Verification items for the finished model (mm, model axes). Round coordinates to 2 decimals unless told otherwise and drop trailing zeros. Write each loop counter-clockwise with the first axis right and the second up, starting at its lowest first coordinate (ties: lowest second). Pieces come first, ordered by that corner, then holes. Notation, with made-up numbers: (31.5, 74.25) - (38.5, 74.25) arc R23 ccw to (38.5, 99.25) - close; hole circle Ø10 at (67, 66). An arc over 180 degrees is marked (long way). Answer as a JSON object with one key per item and string values. Group by question number.
1) Thickness scan on line 1 (Y direction, x = 3, z = 2.25); line 2 (X direction, y = 1.65, z = -2.25); line 3 (Z direction, x = 9.5, y = 0.25). Record the ranges inside material, lowest first.
2) Section check D-D (x = -10). Enter the section's corners in (y, z).
3) Go/stop test with flat-tipped pins: pin 1 Ø4 at (x, z) = (-6, -1.5) entering from +Y; pin 2 Ø3 at (x, z) = (0, 0) entering from +Y. Record where each tip stops, or that it passes through.
4) Section check B-B (y = 0.65). State how many separate pieces and enclosed holes the cut face has, then the cut area to 3 significant figures.
5) Section check A-A (x = 0). Enter the section's corners in (y, z).
6) Section check C-C (z = 0.75). Enter the section's corners in (x, y), then the cut area to 3 significant figures.
```python
from build123d import *
from build123d.topology import SkipClean

# Parameters (mm, degrees)
BOSS_EXTRUDE1_DEPTH = 1.5
SKETCH2_R           = 3.5
BOSS_EXTRUDE2_DEPTH = 2.3
SKETCH3_R           = 0.375
SKETCH3_R_2         = 1.25
CUT_EXTRUDE1_DEPTH  = 17.539044712


with BuildPart() as part:
    # Sketch1 → Boss-Extrude1 (new body)
    with BuildSketch(Plane(origin=(0, 0, 0), x_dir=(1, 0, 0), z_dir=(0, 1, 0))):
        with BuildLine():
            Line((2.257072219, 2.675), (14.110649579, 2))
            ThreePointArc((14.110649579, 2), (16, 0), (14.110649579, -2))
            Line((14.110649579, -2), (2.257072219, -2.675))
            ThreePointArc((2.257072219, -2.675), (-3.5, 0), (2.257072219, 2.675))
        make_face()
    boss_extrude1 = extrude(amount=BOSS_EXTRUDE1_DEPTH)

    # Sketch2 → Boss-Extrude2 (add)
    with SkipClean():  # the faces are left unmerged after this step: merging them gives an invalid solid
        with BuildSketch(Plane(origin=(0, 1.5, 0), x_dir=(1, 0, 0), z_dir=(0, 1, 0))):
            with Locations(Location((0, 0, 0), (0, 0, 49.843487791))):
                Circle(SKETCH2_R)
        extrude(amount=BOSS_EXTRUDE2_DEPTH)

    # Sketch3 → Cut-Extrude1 (cut, symmetric)
    with SkipClean():  # the faces are left unmerged after this step: merging them gives an invalid solid
        with BuildSketch(Plane(origin=(0, 1.5, 0), x_dir=(1, 0, 0), z_dir=(0, 1, 0))):
            with Locations(Location((14.958333333, 0, 0), (0, 0, 270))):
                Circle(SKETCH3_R)
            with Locations(Location((12.875, 0, 0), (0, 0, 270))):
                Circle(SKETCH3_R)
            with Locations(Location((10.791666667, 0, 0), (0, 0, 270))):
                Circle(SKETCH3_R)
            with Locations(Location((8.708333333, 0, 0), (0, 0, 270))):
                Circle(SKETCH3_R)
            with Locations(Location((6.625, 0, 0), (0, 0, 270))):
                Circle(SKETCH3_R)
            with Locations(Location((4.541666667, 0, 0), (0, 0, 270))):
                Circle(SKETCH3_R)
            with Locations(Location((0, 0, 0), (0, 0, 270))):
                Circle(SKETCH3_R_2)
        cut_extrude1 = extrude(amount=CUT_EXTRUDE1_DEPTH, both=True, mode=Mode.SUBTRACT)

    # Mirror1: Boss-Extrude1, Cut-Extrude1 across plane
    with SkipClean():  # the faces are left unmerged after this step: merging them gives an invalid solid
        add(boss_extrude1.mirror(Plane(origin=(0, 0, 0), x_dir=(0, 0, 1), z_dir=(1, 0, 0))))
        add(cut_extrude1.mirror(Plane(origin=(0, 0, 0), x_dir=(0, 0, 1), z_dir=(1, 0, 0))), mode=Mode.SUBTRACT)


solid = part.part
```
Returned:
{
 "1": {"line 1": "0 to 1.5", "line 2": "-2.68 to 2.68", "line 3": "-2.26 to 2.26"},
 "2": {"outline": "(0, -2.23) - (1.5, -2.23) - (1.5, 2.23) - (0, 2.23) - close"},
 "3": {"pin 1": "y = 1.5", "pin 2": "y = 3.8"},
 "4": {"separate pieces": "1", "enclosed holes": "13", "area": "142 mm2"},
 "5": {"outline": "(0, -3.5) - (3.8, -3.5) - (3.8, -1.25) - (0, -1.25) - close; (0, 1.25) - (3.8, 1.25) - (3.8, 3.5) - (0, 3.5) - close"},
 "6": {"outline": "(-15.85, 0) - (-1, 0) - (-1, 3.8) - (-3.42, 3.8) - (-3.42, 1.5) - (-15.85, 1.5) - close; (1, 0) - (15.85, 0) - (15.85, 1.5) - (3.42, 1.5) - (3.42, 3.8) - (1, 3.8) - close", "area": "55.7 mm2"}
}
